Here's how the part is built. I have some questions about the finished solid (model axes, mm). A direction names the side the tool comes from. Give positions to 0.01 mm unless a question says otherwise; leave off trailing zeros. Loops run counter-clockwise (first coordinate to the right, second up) from the corner with the lowest first, then second, coordinate; pieces in that order, holes last.
Q1. Suppose I cut it at B-B (y = 1.5). List the corners of the cut face in (x, z) for me (1 decimal).
Q2. I need wall thicknesses on probe 1 along X at (y, z) = (5.25, -4.25); probe 2 along X at (y, z) = (0.5, 1); probe 3 along X at (y, z) = (3.75, -4.5). Which ranges of each line are inside material? Lowest first, please.
Q3. Thinking about a two-plate mould opening in Z: for faces 6 (the face through (1.923, 5.309, -4.606)), 7 (the face through (2, 3.556, 5)), 8 (the face through (0, 4, -1.714)), which applies, pulls with the +Z half, pulls with the -Z half, needs draft (parallel to the pull), parting line crosses it, or undercut?
Q4. Suppose I cut it at A-A (x = 0). List the corners of the cut face in (y, z) for me (1 decimal).
Q5. I'm going to push flat-ended pins straight in: P1, Ø1.6, axis at x = -2.5, z = 5, coming from the +Y side; P2, Ø0.8, axis at x = 5, y = 4.5, coming from the -Z side; P3, Ø1.6, axis at x = 2, z = 5, coming from the +Y side. Where does each tip first touch, or does it pass through?
Q6. For faces 1 (the face through (1.714, 4, 0)), 2 (the face through (1.897, 5.309, 4.616)), 3 (the face through (-5, 3.556, -2)), 4 (the face through (-2, 3.556, -5)), 5 (the face through (4.606, 5.309, 1.923)), which set-ups out of +Z, -Z, +X, -X, +Y, -Y let a thin tool reach every point of the face, with its end or its side?
```python
from build123d import *

# Parameters (mm, degrees)
SKETCH1_R               = 5.715
BOSS_EXTRUDE2_DEPTH     = 3.556
SKETCH2_R               = 4.990855354
BOSS_EXTRUDE3_DEPTH     = 4.064
SKETCH3_W               = 3.429
SKETCH3_H               = 3.429
CUT_EXTRUDE1_DEPTH      = 1
CUT_EXTRUDE1_DEPTH_BACK = 8.62
FILLET1_R               = 0.508


with BuildPart() as part:
    # Sketch1 → Boss-Extrude2 (new body)
    with BuildSketch(Plane(origin=(0, 0, 0), x_dir=(1, 0, 0), z_dir=(0, 1, 0))):
        Circle(SKETCH1_R)
    extrude(amount=BOSS_EXTRUDE2_DEPTH)

    # Sketch2 → Boss-Extrude3 (add)
    with BuildSketch(Plane(origin=(0, 3.556, 0), x_dir=(1, 0, 0), z_dir=(0, 1, 0))):
        Circle(SKETCH2_R)
        with BuildLine():
            ThreePointArc((0.9779, 5.630713684), (0, 5.715), (-0.9779, 5.630713684))
            Line((-0.9779, 5.630713684), (-0.9779, 4.894113684))
            ThreePointArc((-0.9779, 4.894113684), (0, 4.990855354), (0.9779, 4.894113684))
            Line((0.9779, 4.894113684), (0.9779, 5.630713684))
        make_face()
        with BuildLine():
            Line((-2.769181252, 4.152140695), (-3.290036107, 4.67299555))
            ThreePointArc((-3.290036107, 4.67299555), (-4.041115254, 4.041115254), (-4.67299555, 3.290036107))
            Line((-4.67299555, 3.290036107), (-4.152140695, 2.769181252))
            ThreePointArc((-4.152140695, 2.769181252), (-3.529067664, 3.529067664), (-2.769181252, 4.152140695))
        make_face()
        with BuildLine():
            Line((-4.894113684, 0.9779), (-5.630713684, 0.9779))
            ThreePointArc((-5.630713684, 0.9779), (-5.715, 0), (-5.630713684, -0.9779))
            Line((-5.630713684, -0.9779), (-4.894113684, -0.9779))
            ThreePointArc((-4.894113684, -0.9779), (-4.990855354, 0), (-4.894113684, 0.9779))
        make_face()
        with BuildLine():
            Line((-4.152140695, -2.769181252), (-4.67299555, -3.290036107))
            ThreePointArc((-4.67299555, -3.290036107), (-4.041115254, -4.041115254), (-3.290036107, -4.67299555))
            Line((-3.290036107, -4.67299555), (-2.769181252, -4.152140695))
            ThreePointArc((-2.769181252, -4.152140695), (-3.529067664, -3.529067664), (-4.152140695, -2.769181252))
        make_face()
        with BuildLine():
            Line((-0.9779, -4.894113684), (-0.9779, -5.630713684))
            ThreePointArc((-0.9779, -5.630713684), (0, -5.715), (0.9779, -5.630713684))
            Line((0.9779, -5.630713684), (0.9779, -4.894113684))
            ThreePointArc((0.9779, -4.894113684), (0, -4.990855354), (-0.9779, -4.894113684))
        make_face()
        with BuildLine():
            ThreePointArc((3.290036107, -4.67299555), (4.041115254, -4.041115254), (4.67299555, -3.290036107))
            Line((4.67299555, -3.290036107), (4.152140695, -2.769181252))
            ThreePointArc((4.152140695, -2.769181252), (3.529067664, -3.529067664), (2.769181252, -4.152140695))
            Line((2.769181252, -4.152140695), (3.290036107, -4.67299555))
        make_face()
        with BuildLine():
            ThreePointArc((5.715, 0), (5.693889431, 0.490762823), (5.630713684, 0.9779))
            Line((5.630713684, 0.9779), (4.894113684, 0.9779))
            ThreePointArc((4.894113684, 0.9779), (4.96661105, 0.491336789), (4.990855354, 0))
            ThreePointArc((4.990855354, 0), (4.96661105, -0.491336789), (4.894113684, -0.9779))
            Line((4.894113684, -0.9779), (5.630713684, -0.9779))
            ThreePointArc((5.630713684, -0.9779), (5.693889431, -0.490762823), (5.715, 0))
        make_face()
        with BuildLine():
            ThreePointArc((4.67299555, 3.290036107), (4.041115254, 4.041115254), (3.290036107, 4.67299555))
            Line((3.290036107, 4.67299555), (2.769181252, 4.152140695))
            ThreePointArc((2.769181252, 4.152140695), (3.529067664, 3.529067664), (4.152140695, 2.769181252))
            Line((4.152140695, 2.769181252), (4.67299555, 3.290036107))
        make_face()
    extrude(amount=BOSS_EXTRUDE3_DEPTH)

    # Sketch3 → Cut-Extrude1 (cut, two sides)
    with BuildSketch(Plane(origin=(0, 7.62, 0), x_dir=(1, 0, 0), z_dir=(0, 1, 0))) as cut_extrude1_sk:
        Rectangle(SKETCH3_W, SKETCH3_H)
    extrude(amount=CUT_EXTRUDE1_DEPTH, mode=Mode.SUBTRACT)
    extrude(cut_extrude1_sk.sketch, amount=-CUT_EXTRUDE1_DEPTH_BACK, mode=Mode.SUBTRACT)

    # Fillet1
    fillet1_edges = [part.edges().sort_by_distance(p)[0] for p in [
        (0, 7.62, -1.7145),
        (-1.7145, 7.62, 0),
        (0, 7.62, 1.7145),
        (1.7145, 7.62, 0),
        (1.7145, 0, 0),
        (0, 0, 1.7145),
        (-1.7145, 0, 0),
        (0, 0, -1.7145),
        (-5.715, 0, 0),
        (-0.9779, 7.62, 5.262413684),
        (0.9779, 7.62, 5.262413684),
        (1.909917657, 7.62, 4.610949111),
        (4.041115254, 7.62, 4.041115254),
        (4.412568123, 7.62, 3.02960868),
        (4.610949111, 7.62, 1.909917657),
        (5.715, 7.62, 0),
        (5.262413684, 7.62, -0.9779),
        (4.610949111, 7.62, -1.909917657),
        (4.041115254, 7.62, -4.041115254),
        (3.02960868, 7.62, -4.412568123),
        (1.909917657, 7.62, -4.610949111),
        (0, 7.62, -5.715),
        (-0.9779, 7.62, -5.262413684),
        (-1.909917657, 7.62, -4.610949111),
        (-4.041115254, 7.62, -4.041115254),
        (-4.412568123, 7.62, -3.02960868),
        (-4.610949111, 7.62, -1.909917657),
        (-5.715, 7.62, 0),
        (-5.262413684, 7.62, 0.9779),
        (-4.610949111, 7.62, 1.909917657),
        (-4.041115254, 7.62, 4.041115254),
        (-3.02960868, 7.62, 4.412568123),
        (-1.909917657, 7.62, 4.610949111),
        (0, 7.62, 5.715),
        (3.02960868, 7.62, 4.412568123),
        (5.262413684, 7.62, 0.9779),
        (4.412568123, 7.62, -3.02960868),
        (0.9779, 7.62, -5.262413684),
        (-3.02960868, 7.62, -4.412568123),
        (-5.262413684, 7.62, -0.9779),
        (-4.412568123, 7.62, 3.02960868),
    ]]
    fillet(fillet1_edges, radius=FILLET1_R)


solid = part.part
```
Solutions:
1. outline: circle Ø11.4 at (0, 0); hole (-1.7, -1.7) - (1.7, -1.7) - (1.7, 1.7) - (-1.7, 1.7) - close
2. probe 1: x = -3.82 to -2.87, -2.62 to 2.62, 2.87 to 3.82
2. probe 2: x = -5.63 to -1.71, 1.71 to 5.63
2. probe 3: x = -3.52 to -3.12, -2.16 to 2.16, 3.12 to 3.52
3. face 6: pulls with the -Z half
3. face 7: needs draft
3. face 8: undercut
4. outline: (0, -5.2) arc R0.5 ccw to (0.5, -5.7) - (7.1, -5.7) arc R0.5 ccw to (7.6, -5.2) - (7.6, -2.2) arc R0.5 ccw to (7.1, -1.7) - (0.5, -1.7) arc R0.5 ccw to (0, -2.2) - close; (0, 2.2) arc R0.5 ccw to (0.5, 1.7) - (7.1, 1.7) arc R0.5 ccw to (7.6, 2.2) - (7.6, 5.2) arc R0.5 ccw to (7.1, 5.7) - (0.5, 5.7) arc R0.5 ccw to (0, 5.2) - close
5. P1: stops at y = 7.52
5. P2: stops at z = -3.39
5. P3: stops at y = 7.61
6. face 1: +Y, -Y
6. face 2: +Z, +Y
6. face 3: -X, +Y
6. face 4: -Z, +Y
6. face 5: +X, +Y
